CAD build for the part. Positions are in the model's coordinates, mm. Face numbers are marked on the shaded views. Coordinates: 2 decimals unless noted, no trailing zeros. Loops run counter-clockwise (first coordinate to the right, second up) from the corner with the lowest first, then second, coordinate; pieces in that order, holes last. Notation, with made-up numbers: (59, 32.5) -> (63, 32.5) arc R22 ccw to (63, 41.5) -> close; hole circle Ø2 at (89, -19.75). An arc over 180 degrees is marked (long way). Return JSON: item names as keys, results as strings. Group by question number.
(1) Mould opens along X. For the marked faces 1 and 2 say: pulls with the +X half, pulls with the -X half, needs draft (parallel to the pull), parting line crosses it, or undercut.
(2) Saw through at D-D on z = -450.5. Write the cut outline in (x, y).
(3) Saw through at C-C on z = -373.5. Write the cut outline in (x, y), then the cut area to 3 significant figures.
(4) Saw through at A-A on z = -114.5. Write the cut outline in (x, y).
(5) Probe L1, parallel to Z at x = 64, y = 16; L2, parallel to X at y = 16.8, z = -411.4; L3, parallel to Z at x = 63, y = 10. List the from-to ranges inside material, lowest first.
(6) Saw through at B-B on z = -295.5. Write the cut outline in (x, y), then the cut area to 3 significant figures.
(7) Flat gauge pins, fed straight in: pin 1 Ø1 at (x, z) = (87.5, -381) entering from +Y; pin 2 Ø6.5 at (x, y) = (125, 22) entering from +Z; pin 3 Ø14.5 at (x, z) = (126.74, -295.5) entering from -Y; pin 4 Ø1.8 at (x, y) = (5.5, 22.5) entering from +Z. Where does each tip first touch, or does it go through?
Autodesk Inventor part; units mm, degrees
ref_plane "YZ Plane" through (0, 0, 0) normal (1, 0, 0) x (0, 1, 0)
ref_plane "XZ Plane" through (0, 0, 0) normal (0, 1, 0) x (-1, 0, 0)
ref_plane "XY Plane" through (0, 0, 0) normal (0, 0, 1) x (1, 0, 0)
sketch "Sketch1" plane through (0, 0, 0) normal (0, 0, 1) x (1, 0, 0)
  line L0 (-7.7614, 0) -> (138.2386, 0)
  line L1 (138.2386, 0) -> (138.2386, 29.6)
  line L2 (-7.7614, 29.6) -> (-7.7614, 0)
  line L3 (-7.7614, 29.6) -> (22.1386, 29.6)
  line L4 (12.489, 18.1) -> (114.8883, 18.1)
  line L5 (22.1386, 29.6) -> (12.489, 18.1)
  line L6 (22.1386, 29.6) -> (41.4586, 29.6) construction
  line L7 (138.2386, 29.6) -> (105.2386, 29.6)
  line L8 (105.2386, 29.6) -> (114.8883, 18.1)
  point P0 (0, 0)
  dimension "d0" = 146
  dimension "d1" = 29.6
  dimension "d2" = 29.9
  dimension "d4" = 130
  dimension "d5" = 33
  dimension "d6" = 50
extrude "Extrusion1" add sketch "Sketch1" against normal blind 486
sketch "Sketch2" plane through (-7.7614, 29.6, 0) normal (0, 1, 0) x (1, 0, 0)
  line L0 (113, 0) -> (122.6496, 0)
  line L1 (124, 486) -> (113, 0)
  line L2 (113, 0) -> (113, 486)
  line L3 (113, 486) -> (124, 486)
  line L4 (122.6496, 0) -> (122.6496, 486)
  line L5 (113, 486) -> (113, 0)
  line L6 (146, 0) -> (146, 486)
  point P0 (7.7614, 0)
  dimension "d9" = 22
sketch "Sketch3" plane through (-7.7614, 0, 0) normal (0, -1, 0) x (1, 0, 0)
  line L0 (20.2504, -486) -> (122.6496, -486)
  line L1 (0, 0) -> (146, 0)
  circle A0 centre (71.6943, -409.4001) radius 62.1
  line L2 (71.45, -486) -> (71.4962, -471.5001)
  circle A1 centre (71.6943, -409.4001) radius 52
  circle A2 centre (71.6943, -409.4001) radius 9.51
  circle A3 centre (72.1613, -247.2004) radius 4.1
  point P0 (7.7614, 0)
  dimension "d10" = 124.2
  dimension "d11" = 14.5
  dimension "d12" = 62.1
  dimension "d13" = 104
  dimension "d14" = 19.02
  dimension "d15" = 8.2
extrude "Extrusion2" cut sketch "Sketch3" against normal blind 13 contours A0
extrude "Extrusion3" add sketch "Sketch3" along normal blind 7.5 contours A2
extrude "Extrusion4" cut sketch "Sketch3" against normal through all contours A3
sketch "Sketch4" plane through (12.489, 18.1, 0) normal (0, 1, 0) x (1, 0, 0)
  circle A0 centre (51.911, 247.2004) radius 4.1
  circle A1 centre (51.911, 247.2004) radius 9.5
  line L0 (0, 486) -> (102.3993, 486)
  line L1 (51.1996, 486) -> (51.1996, 476.6)
  arc A2 (46.6496, 476.6) -> (46.6496, 457.9) centre (46.6496, 467.25) ccw
  arc A3 (55.7496, 457.9) -> (55.7496, 476.6) centre (55.7496, 467.25) ccw
  line L2 (46.6496, 476.6) -> (55.7496, 476.6)
  line L3 (46.6496, 457.9) -> (55.7496, 457.9)
  circle A4 centre (51.1996, 411.4) radius 8.5
  point P0 (-12.489, 0)
  point P1 (51.1996, 476.6)
  dimension "d23" = 19
  dimension "d26" = 9.4
  dimension "d29" = 0
  dimension "d30" = 18.7
  dimension "d31" = 18.7
  dimension "d38" = 17
  dimension "d39" = 46.5
extrude "Extrusion5" cut sketch "Sketch4" against normal blind 3.7 contours A1
extrude "Extrusion7" cut sketch "Sketch4" against normal blind 6 contours L2 A3 L3 A2
extrude "Extrusion8" cut sketch "Sketch4" against normal blind 3 contours A4
sketch "Sketch5" plane through (-7.7614, 0, 0) normal (0, -1, 0) x (1, 0, 0)
  point P0 (7.7614, 0)
sketch "Sketch6" plane through (-7.7614, 0, 0) normal (0, -1, 0) x (1, 0, 0)
  circle A0 centre (86, -261) radius 5
  line L0 (146, -486) -> (0, -486)
  line L1 (146, 0) -> (146, -486)
  circle A1 centre (60.5, -235.5) radius 5.5
  line L2 (0, 0) -> (0, -486)
  circle A2 centre (134.5, -295.5) radius 5.5
  point P0 (7.7614, 0)
  dimension "d42" = 10
  dimension "d43" = 225
  dimension "d44" = 60
  dimension "d45" = 11
  dimension "d46" = 60.5
  dimension "d47" = 250.5
  dimension "d48" = 11
  dimension "d49" = 190.5
  dimension "d50" = 11.5
hole "Hole1" at (126.7386, 0, -295.5) direction (0, 1, 0) diameter 8.5 end through all counterbore diameter 11 counterbore depth 8.5
hole "Hole2" at (78.2386, 0, -261) direction (0, 1, 0) diameter 7 end through all counterbore diameter 10 counterbore depth 7.5
hole "Hole3" at (52.7386, 0, -235.5) direction (0, 1, 0) diameter 7.5 end through all counterbore diameter 11 counterbore depth 7
thread "Thread1"
sketch "Sketch12" plane through (0, 0, 0) normal (0, 0, 1) x (1, 0, 0)
  circle A0 centre (125.0477, 23) radius 3
  circle A1 centre (100.0477, 8) radius 3
  circle A2 centre (30.0477, 8) radius 3
  circle A3 centre (5.0477, 23) radius 3
  circle A4 centre (67.1736, 14.602) radius 2.25
  point P0 (0, 0)
extrude "Extrusion9" cut sketch "Sketch12" against normal blind 20
properties part number "slide ontop of saddle" material "Steel, Cast"
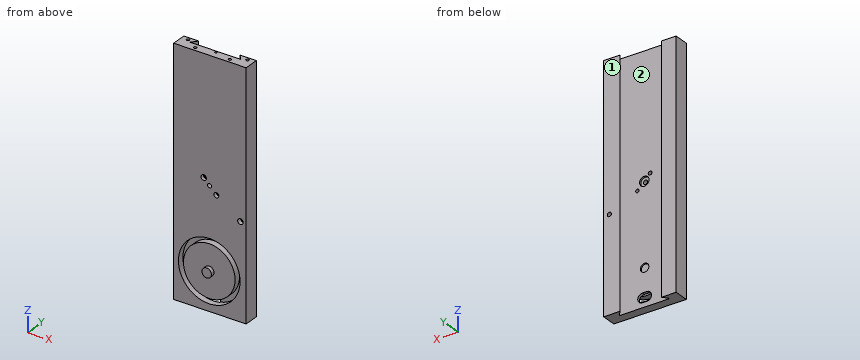
Geometry results:
{
 "1": {"face 1": "needs draft", "face 2": "undercut"},
 "2": {"outline": "(-7.76, 0) -> (17.38, 0) -> (17.38, 13) -> (32.08, 13) -> (32.08, 0) -> (95.79, 0) -> (95.79, 13) -> (110.49, 13) -> (110.49, 0) -> (138.24, 0) -> (138.24, 29.6) -> (105.24, 29.6) -> (114.89, 18.1) -> (12.49, 18.1) -> (22.14, 29.6) -> (-7.76, 29.6) -> close"},
 "3": {"outline": "(-7.76, 0) -> (13.26, 0) -> (13.26, 13) -> (26.31, 13) -> (26.31, 0) -> (101.55, 0) -> (101.55, 13) -> (114.6, 13) -> (114.6, 0) -> (138.24, 0) -> (138.24, 29.6) -> (105.24, 29.6) -> (114.89, 18.1) -> (12.49, 18.1) -> (22.14, 29.6) -> (-7.76, 29.6) -> close", "area": "2,920 mm²"},
 "4": {"outline": "(-7.76, 0) -> (138.24, 0) -> (138.24, 29.6) -> (105.24, 29.6) -> (114.89, 18.1) -> (12.49, 18.1) -> (22.14, 29.6) -> (-7.76, 29.6) -> close"},
 "5": {"L1": "-486 to -476.6, -457.9 to -419.89, -402.91 to -256.69, -237.71 to 0", "L2": "-7.76 to 55.19, 72.19 to 138.24", "L3": "-486 to -471.49, -461.39 to -357.41, -347.31 to -251.05, -243.35 to 0"},
 "6": {"outline": "(-7.76, 0) -> (121.24, 0) -> (121.24, 8.5) -> (122.49, 8.5) -> (122.49, 29.6) -> (105.24, 29.6) -> (114.89, 18.1) -> (12.49, 18.1) -> (22.14, 29.6) -> (-7.76, 29.6) -> close; (130.99, 8.5) -> (132.24, 8.5) -> (132.24, 0) -> (138.24, 0) -> (138.24, 29.6) -> (130.99, 29.6) -> close", "area": "2,980 mm²"},
 "7": {"pin 1": "y = 18.1", "pin 2": "z = 0", "pin 3": "y = 0", "pin 4": "z = -20"}
}
